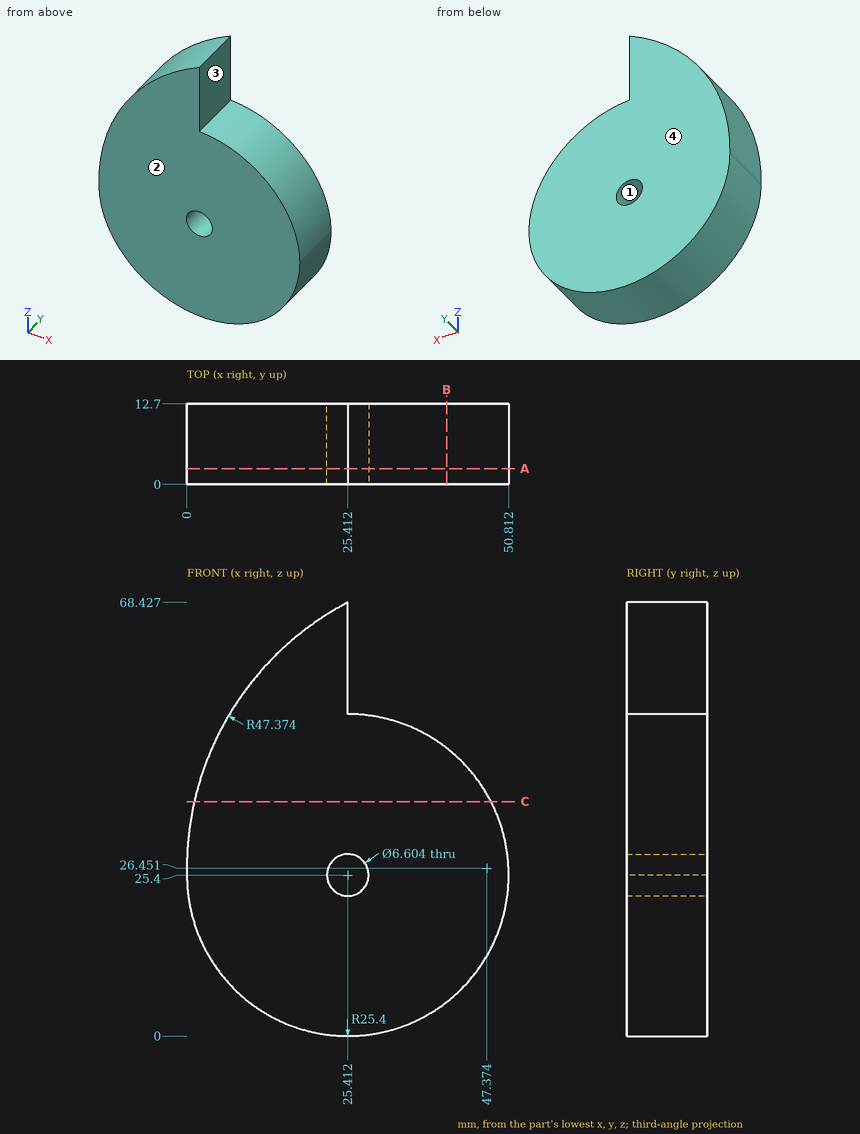
Input: dimensioned drawing with shaded views. Units: mm. Origin: part minimum x, y, z. A direction names the side the tool comes from. Coordinates: 2 decimals unless noted, no trailing zeros. Order: outer loops, then holes, each group sorted by start corner. A loop starts at its lowest first (then second) coordinate and runs counter-clockwise, first axis right, second up.
Item 1: Section query A-A (y = 2.5). Output: boundary loops of the cut face in (x, z).
Answer:
outline: (0.01, 25.4) arc R25.4 ccw (long way) to (25.41, 50.8) - (25.41, 68.43) arc R47.37 ccw to start; hole circle Ø6.6 at (25.41, 25.4)
Item 2: Access query for the marked faces 3 and 4. Directions: +Z, -Z, +X, -X, +Y, -Y. A direction counts if a zero-diameter tool reaches every point of the face in a straight line with its end or side. Return the directions, or none.
Answer:
face 3: +Z, +X, +Y, -Y
face 4: +Z, -Z, +X, -X, +Y
Item 3: Draft query along Z for the marked faces 1 and 2. Return one class per face: released by +Z, released by -Z, zero draft, split by the parting line, or undercut.
Answer:
face 1: undercut
face 2: zero draft
Item 4: Contact query for flat-ended pins moving along their axis: P1, Ø3, axis at y = 3.5, z = 31, coming from the +X side; P2, Ø3, axis at x = 14, y = 8, coming from the +Z side; P3, Ø2, axis at y = 5, z = 10.5, coming from the +X side. Output: stop coordinate, or through.
Answer:
P1: stops at x = 50.48
P2: stops at z = 61.5
P3: stops at x = 46.67
Item 5: Material intervals for line 1 along X through (y, z) = (9.25, 61); line 2 along Z through (x, y) = (17.5, 6) (1 decimal); line 3 along Z through (x, y) = (35, 6.25), sorted ascending.
Answer:
line 1: x = 14.96 to 25.41
line 2: z = 1.3 to 63.2
line 3: z = 1.88 to 48.92
Item 6: Section query C-C (z = 37). Output: boundary loops of the cut face in (x, y), then the cut area to 3 significant figures.
Answer:
outline: (1.19, 0) - (48.01, 0) - (48.01, 12.7) - (1.19, 12.7) - close
area: 595 mm2
Item 7: Section query B-B (x = 41). Output: boundary loops of the cut face in (y, z).
Answer:
outline: (0, 5.35) - (12.7, 5.35) - (12.7, 45.45) - (0, 45.45) - close
